Check sheet for the modelled part. Datum: model origin and axes. Units: mm. A direction names the side the tool comes from. Give positions to 0.01 mm unless a question says otherwise; leave off trailing zeros. Order: outer loops, then holes, each group sorted by start corner. A loop starts at its lowest first (then second) coordinate and runs counter-clockwise, first axis right, second up.
Item 1: Sectioned sample at A-A on x = 10. Record the boundary of the cut face in (y, z), and give its area (3 significant figures).
Item 2: Release check for a two-part mould opening along Z. For faces 1 (the flat face through (20, -4, 4)), 2 (the flat face through (26, -42, -88)), 3 (the flat face through (0.055, 23, -134)), 4 (the flat face through (26, -40, -97)) record: released by +Z, released by -Z, zero draft, split by the parting line, or undercut.
Item 3: Material ranges on line 1 along Y through (x, z) = (10, 1.8); line 2 along Z through (x, y) = (30, 4.5); line 3 along Y through (x, z) = (14, -101.5), recorded low to high.
Item 4: Gauge pin test, flat ends, axial feed: P1, Ø2, axis at x = 3, z = -134.5, coming from the -Y side; P2, Ø12, axis at y = -34.5, z = -78, coming from the -X side; P3, Ø4.5, axis at y = -7, z = 2, coming from the -X side. Record the tip position at first contact, or that the pin passes through.
Item 5: Sectioned sample at C-C on x = 22. Record the boundary of the cut face in (y, z), and give its area (3 significant figures).
Item 6: Access from +Z, -Z, +X, -X, +Y, -Y to the whole of each face (thin tool, end or side, straight path). Record for faces 5 (the flat face through (22, -43, -6)), 6 (the flat face through (22, -49, -20)), 7 (the flat face through (26, -42, -107)).
Item 7: Sectioned sample at B-B on y = -21. Record the boundary of the cut face in (x, z).
Item 8: Sectioned sample at D-D on y = 23. Record the boundary of the cut face in (x, z).
from build123d import *

# Parameters (mm, degrees)
SKETCH010_W   = 12
SKETCH010_H   = 19
PAD004_DEPTH  = 3
SKETCH003_W   = 20
SKETCH003_H   = 5
PAD001_DEPTH  = 132
PAD002_DEPTH  = 4
SKETCH005_R   = 3.3
HOLE001_DEPTH = 4.001
SKETCH006_W   = 20
SKETCH006_H   = 4
PAD003_DEPTH  = 24
SKETCH009_R   = 6.6
HOLE002_DEPTH = 4.001
PAD_DEPTH     = 4
SKETCH002_R   = 3.3
HOLE_DEPTH    = 4.001


with BuildPart() as body004:
    # Sketch010 (on Face1 of CopyPad001001) → Pad004 (new body)
    with BuildSketch(Plane.XZ.offset(43)):
        with Locations((26, -97.5)):
            Rectangle(SKETCH010_W, SKETCH010_H)
    extrude(amount=-PAD004_DEPTH)


with BuildPart() as body001:
    # Sketch003 (on Face1 of CopyHole) → Pad001 (new body)
    with BuildSketch(Plane(origin=(0, 0, 0), x_dir=(1, 0, 0), z_dir=(0, 0, -1))):
        with Locations((22, 40.5)):
            Rectangle(SKETCH003_W, SKETCH003_H)
    extrude(amount=PAD001_DEPTH)

    # Boolean: cut Body004
    add(body004.part, mode=Mode.SUBTRACT)


with BuildPart() as body002:
    # Sketch004 → Pad002 (new body)
    with BuildSketch(Plane.XY):
        Polygon((0.055073, 33), (32.055073, 33), (32.055073, -43), (12.055073, -43), (12.055073, 13), (0.055073, 13), align=None)
    extrude(amount=PAD002_DEPTH)

    # Sketch005 (on Face8 of Pad002) → Hole001 (cut, through all)
    with BuildSketch(Plane.XY.offset(4)):
        with Locations((10, 23)):
            Circle(SKETCH005_R)
    extrude(amount=-HOLE001_DEPTH, mode=Mode.SUBTRACT)


with BuildPart() as body002_1:
    # Body002 placement: moved
    add(body002.part.moved(Location((0, 0, -136))))


with BuildPart() as body003:
    # Sketch006 (on Face1 of CopyPad001) → Pad003 (new body)
    with BuildSketch(Plane.XZ.offset(43)):
        with Locations((22, -18)):
            Rectangle(SKETCH006_W, SKETCH006_H)
    extrude(amount=PAD003_DEPTH)

    # Sketch009 (on Face1 of Pad003) → Hole002 (cut, through all)
    with BuildSketch(Plane.XY.offset(-16)):
        with Locations((22, -58)):
            Circle(SKETCH009_R)
    extrude(amount=-HOLE002_DEPTH, mode=Mode.SUBTRACT)


with BuildPart() as body:
    # Sketch → Pad (new body)
    with BuildSketch(Plane.XY):
        Polygon((0.055073, 33), (32.055073, 33), (32.055073, -43), (12.055073, -43), (12.055073, 13), (0.055073, 13), align=None)
    extrude(amount=PAD_DEPTH)

    # Sketch002 (on Face8 of Pad) → Hole (cut, through all)
    with BuildSketch(Plane.XY.offset(4)):
        with Locations((10, 23)):
            Circle(SKETCH002_R)
    extrude(amount=-HOLE_DEPTH, mode=Mode.SUBTRACT)

    # Boolean001: union Body001
    add(body001.part)

    # Boolean002: union Body002
    add(body002_1.part)

    # Boolean003: union Body003
    add(body003.part)


solid = body.part
Report:
1. outline: (13, -136) - (19.7, -136) - (19.7, -132) - (13, -132) - close; (13, 0) - (19.7, 0) - (19.7, 4) - (13, 4) - close; (26.3, -136) - (33, -136) - (33, -132) - (26.3, -132) - close; (26.3, 0) - (33, 0) - (33, 4) - (26.3, 4) - close
1. area: 107 mm2
2. face 1: released by +Z
2. face 2: undercut
2. face 3: zero draft
2. face 4: undercut
3. line 1: y = 13 to 19.7, 26.3 to 33
3. line 2: z = -136 to -132, 0 to 4
3. line 3: y = -43 to -38
4. P1: stops at y = 13
4. P2: stops at x = 12
4. P3: stops at x = 12.06
5. outline: (-67, -20) - (-64.6, -20) - (-64.6, -16) - (-67, -16) - close; (-51.4, -20) - (-43, -20) - (-43, -88) - (-40, -88) - (-40, -107) - (-43, -107) - (-43, -136) - (33, -136) - (33, -132) - (-38, -132) - (-38, 0) - (33, 0) - (33, 4) - (-43, 4) - (-43, -16) - (-51.4, -16) - close
5. area: 1,250 mm2
6. face 5: +Z, +X, -X, -Y
6. face 6: -Z, +X, -X, -Y
6. face 7: +X, -Y
7. outline: (12.06, -136) - (32.06, -136) - (32.06, -132) - (12.06, -132) - close; (12.06, 0) - (32.06, 0) - (32.06, 4) - (12.06, 4) - close
8. outline: (0.06, -136) - (6.7, -136) - (6.7, -132) - (0.06, -132) - close; (0.06, 0) - (6.7, 0) - (6.7, 4) - (0.06, 4) - close; (13.3, -136) - (32.06, -136) - (32.06, -132) - (13.3, -132) - close; (13.3, 0) - (32.06, 0) - (32.06, 4) - (13.3, 4) - close
